The listing builds one solid part. Answer for the finished solid, in the listing's coordinates (mm). Face numbers are marked on the shaded views. A direction names the side the tool comes from. Give positions to 0.01 mm unless a question says otherwise; leave off trailing zeros. Loops run counter-clockwise (first coordinate to the right, second up) from the corner with the lowest first, then second, coordinate; pieces in that order, holes last. Notation, with made-up numbers: M 10,13.25 L 14,13.25 A19 cw 14,43.25 Z; hole C 14.25,0 d2. An arc over 180 degrees is marked long. One line per item, written item: value. Start each with the question number.
Q1. Consider L1, parallel to X at y = -1, z = 0; L2, parallel to Z at x = -12, y = -24; L3, parallel to X at y = -4, z = -15.5. Determine where each line is inside the solid, lowest interval first.
Q2. The mould has two halves that part along Z. Classify the marked faces 4, 5, 6 and 7: +Z half, -Z half, draft (parallel to the pull), parting line (faces both ways), or undercut.
Q3. A cutting plane is placed at D-D, the plane x = -8. Determine the outline of the cut face in (y, z).
Q4. A cutting plane is placed at B-B, the plane y = -23.25. Determine the outline of the cut face in (x, z).
Q5. Flat-ended cylindrical pins translate along their axes: pin 1 (2 mm diameter, centred on x = 8, z = 0, fed in from -Y); pin 2 (5 mm diameter, centred on x = 10.5, y = -31.5, fed in from -Z); pin 3 (15.5 mm diameter, centred on x = 3.5, y = -20, fed in from +Z); pin 4 (6 mm diameter, centred on x = -11.5, z = 2.5, fed in from -Y). Find the tip coordinate at first contact, or state that the pin passes through.
Q6. For the marked faces 1, 2 and 3, determine the directions among +Z, -Z, +X, -X, +Y, -Y from which every point of the face is accessible in a straight line to the end or side of a thin tool.
Q7. A cutting plane is placed at C-C, the plane z = 23. Determine the outline of the cut face in (x, y), and give its area (3 significant figures).
Q8. A cutting plane is placed at A-A, the plane z = 0. Determine the outline of the cut face in (x, y).
from build123d import *

# Parameters (mm, degrees)
SKETCH1_W               = 41
SKETCH1_H               = 96
SKETCH1_R               = 4
SKETCH1_R_2             = 1.85
BOSS_EXTRUDE1_DEPTH     = 43.5
CUT_EXTRUDE1_DEPTH      = 108.370852656
CUT_EXTRUDE1_DEPTH_BACK = 26
CUT_EXTRUDE2_START      = -96
CUT_EXTRUDE2_DEPTH      = 26
SKETCH4_W               = 41
SKETCH4_H               = 38
CUT_EXTRUDE4_DEPTH      = 40.5
BOSS_EXTRUDE2_START     = 20.5
BOSS_EXTRUDE2_DEPTH     = 5
BOSS_EXTRUDE3_START     = -15.5
BOSS_EXTRUDE3_DEPTH     = 5
CUT_EXTRUDE5_START      = -44
CUT_EXTRUDE5_DEPTH      = 44


# Read off the part's stored shape, not the designer's step: Cut-Extrude5
with BuildPart() as part:
    # Sketch1 → Boss-Extrude1 (new body)
    with BuildSketch(Plane(origin=(0, 0, 0), x_dir=(1, 0, 0), z_dir=(0, 1, 0))):
        Rectangle(SKETCH1_W, SKETCH1_H)
        with Locations(Location((0, 0, 0), (0, 0, 270))):
            Circle(SKETCH1_R, mode=Mode.SUBTRACT)
        with Locations(Location((0, -8, 0), (0, 0, 270))):
            Circle(SKETCH1_R_2, mode=Mode.SUBTRACT)
        with Locations(Location((-8, 0, 0), (0, 0, 270))):
            Circle(SKETCH1_R_2, mode=Mode.SUBTRACT)
        with Locations(Location((0, 8, 0), (0, 0, 270))):
            Circle(SKETCH1_R_2, mode=Mode.SUBTRACT)
        with Locations(Location((8, 0, 0), (0, 0, 270))):
            Circle(SKETCH1_R_2, mode=Mode.SUBTRACT)
    extrude(amount=-BOSS_EXTRUDE1_DEPTH)

    # Sketch3 → Cut-Extrude1 (cut, two sides: drawn at the far end of the back side and taken through both)
    with BuildSketch(Plane.XY.offset(48).offset(-CUT_EXTRUDE1_DEPTH_BACK)):
        with BuildLine():
            Line((-18.340899032, -19.35462804), (-20.5, -21.513729008))
            Line((-20.5, -21.513729008), (-20.5, -43.5))
            Line((-20.5, -43.5), (2.768563004, -43.5))
            Line((2.768563004, -43.5), (4.927663972, -41.340899032))
            ThreePointArc((4.927663972, -41.340899032), (12.877412268, -9.621546189), (-18.340899032, -19.35462804))
        make_face()
    extrude(amount=CUT_EXTRUDE1_DEPTH + CUT_EXTRUDE1_DEPTH_BACK, mode=Mode.SUBTRACT)

    # Sketch3<4> → Cut-Extrude2 (cut)
    with BuildSketch(Plane.XY.offset(48).offset(CUT_EXTRUDE2_START)):
        with BuildLine():
            Line((-18.340899032, -19.35462804), (-20.5, -21.513729008))
            Line((-20.5, -21.513729008), (-20.5, -43.5))
            Line((-20.5, -43.5), (2.768563004, -43.5))
            Line((2.768563004, -43.5), (4.927663972, -41.340899032))
            ThreePointArc((4.927663972, -41.340899032), (12.877412268, -9.621546189), (-18.340899032, -19.35462804))
        make_face()
    extrude(amount=CUT_EXTRUDE2_DEPTH, mode=Mode.SUBTRACT)

    # Sketch4 → Cut-Extrude4 (cut)
    with BuildSketch(Plane.XZ.offset(43.5)):
        Rectangle(SKETCH4_W, SKETCH4_H)
    extrude(amount=-CUT_EXTRUDE4_DEPTH, mode=Mode.SUBTRACT)

    # Sketch5 → Boss-Extrude2 (add)
    with BuildSketch(Plane(origin=(0, 0, 0), x_dir=(0, 0, -1), z_dir=(1, 0, 0)).offset(BOSS_EXTRUDE2_START)):
        with BuildLine():
            Line((-19, -43.5), (-3.646281893, -27.13616886))
            ThreePointArc((-3.646281893, -27.13616886), (0, -25.557371624), (3.646281893, -27.13616886))
            Line((3.646281893, -27.13616886), (19, -43.5))
            Line((19, -43.5), (19, -3))
            Line((19, -3), (-19, -3))
            Line((-19, -3), (-19, -43.5))
        make_face()
    extrude(amount=-BOSS_EXTRUDE2_DEPTH)

    # Sketch5<2> → Boss-Extrude3 (add)
    with BuildSketch(Plane(origin=(0, 0, 0), x_dir=(0, 0, -1), z_dir=(1, 0, 0)).offset(BOSS_EXTRUDE3_START)):
        with BuildLine():
            Line((-19, -43.5), (-3.646281893, -27.13616886))
            ThreePointArc((-3.646281893, -27.13616886), (0, -25.557371624), (3.646281893, -27.13616886))
            Line((3.646281893, -27.13616886), (19, -43.5))
            Line((19, -43.5), (19, -3))
            Line((19, -3), (-19, -3))
            Line((-19, -3), (-19, -43.5))
        make_face()
    extrude(amount=-BOSS_EXTRUDE3_DEPTH)

    # Cut-Extrude5 outline → Cut-Extrude5 (cut)
    with BuildSketch(Plane.XY.offset(22).offset(CUT_EXTRUDE5_START)):
        with BuildLine():
            Line((-20.5, -43.5), (-2.768563004, -43.5))
            ThreePointArc((-2.768563004, -43.5), (-14.946344874, -37.246752593), (-20.5, -24.734423107))
            Line((-20.5, -24.734423107), (-20.5, -43.5))
        make_face()
    extrude(amount=CUT_EXTRUDE5_DEPTH, mode=Mode.SUBTRACT)


solid = part.part
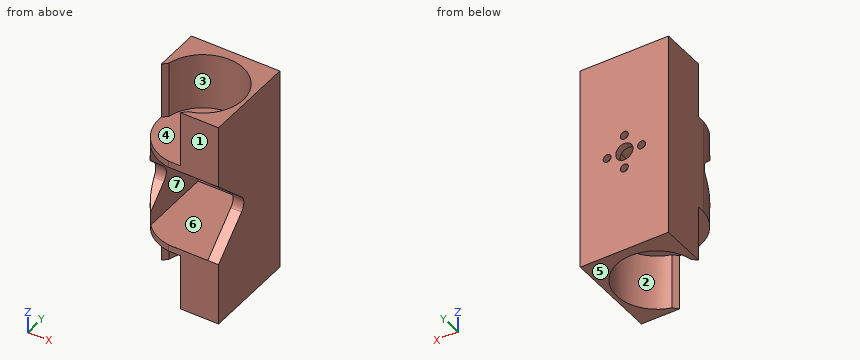
Answer block:
1. L1: -20.5 to -9.85, -6.15 to -4, 4 to 6.15, 9.85 to 20.5
1. L2: -22 to -19, 19 to 22
1. L3: -20.5 to -15.5, 15.5 to 20.5
2. face 4: +Z half
2. face 5: -Z half
2. face 6: undercut
2. face 7: undercut
3. outline: M -42.07,-22 L -6.29,-22 L -6.29,-48 L 0,-48 L 0,-1.85 L -3,-1.85 L -3,-19 L -42.07,-19 Z; M -42.07,19 L -3,19 L -3,1.85 L 0,1.85 L 0,48 L -6.29,48 L -6.29,22 L -42.07,22 Z
4. outline: M -20.5,-22 L 18.75,-22 L 18.75,-48 L 20.5,-48 L 20.5,48 L 18.75,48 L 18.75,22 L -20.5,22 Z; hole M -15.5,-19 L 15.5,-19 L 15.5,19 L -15.5,19 Z
5. pin 1: through
5. pin 2: z = -22
5. pin 3: z = 22
5. pin 4: y = -3
6. face 1: +Z, -Z, +X, -X, -Y
6. face 2: -Z
6. face 3: +Z
7. outline: M -20.5,-21.51 L -18.34,-19.35 A18.75 cw long 4.93,-41.34 L 2.77,-43.5 L 20.5,-43.5 L 20.5,0 L -20.5,0 Z
7. area: 529 mm^2
8. outline: M -20.5,-24.73 A20.56 ccw -20.42,-25.56 L -15.5,-25.56 L -15.5,-3 L -9.85,-3 L -9.85,0 L -20.5,0 Z; M -6.15,-3 L -4,-3 L -4,0 L -6.15,0 Z; M 4,-3 L 6.15,-3 L 6.15,0 L 4,0 Z; M 9.85,-3 L 15.5,-3 L 15.5,-25.56 L 20.5,-25.56 L 20.5,0 L 9.85,0 Z
